```python
from build123d import *

# Parameters (mm, degrees)
SKETCH1_W           = 147.32
SKETCH1_H           = 93.98
SKETCH1_W_2         = 139.7
SKETCH1_H_2         = 86.36
BOSS_EXTRUDE1_DEPTH = 30.48
SKETCH2_W           = 147.32
SKETCH2_H           = 93.98
BOSS_EXTRUDE2_DEPTH = 3.81
FILLET1_R           = 7.62
FILLET2_R           = 5.08
CUT_EXTRUDE2_REACH  = 95.86
SKETCH4_W           = 105.5116
SKETCH4_H           = 67.2084
CUT_EXTRUDE3_REACH  = 94.536
SKETCH5_R           = 2.58


with BuildPart() as part:
    # Sketch1 → Boss-Extrude1 (new body)
    with BuildSketch(Plane(origin=(0, 0, 0), x_dir=(1, 0, 0), z_dir=(0, 1, 0))):
        Rectangle(SKETCH1_W, SKETCH1_H)
        Rectangle(SKETCH1_W_2, SKETCH1_H_2, mode=Mode.SUBTRACT)
    extrude(amount=BOSS_EXTRUDE1_DEPTH)

    # Sketch2 → Boss-Extrude2 (add)
    with BuildSketch(Plane(origin=(0, 0, 0), x_dir=(-1, 0, 0), z_dir=(0, -1, 0))):
        Rectangle(SKETCH2_W, SKETCH2_H)
    extrude(amount=BOSS_EXTRUDE2_DEPTH)

    # Fillet1
    fillet1_edges = [part.edges().sort_by_distance(p)[0] for p in [
        (-73.66, 13.335, -46.99),
        (73.66, 13.335, -46.99),
        (73.66, 13.335, 46.99),
        (-73.66, 13.335, 46.99),
    ]]
    fillet(fillet1_edges, radius=FILLET1_R)

    # Fillet2
    fillet2_edges = [part.edges().sort_by_distance(p)[0] for p in [
        (-69.85, 15.24, -43.18),
        (-69.85, 15.24, 43.18),
        (69.85, 15.24, 43.18),
        (69.85, 15.24, -43.18),
    ]]
    fillet(fillet2_edges, radius=FILLET2_R)

    # Sketch4 → Cut-Extrude2 (cut, up to next)
    with BuildSketch(Plane.XZ.offset(3.81), mode=Mode.PRIVATE) as cut_extrude2_sk1:
        Rectangle(SKETCH4_W, SKETCH4_H)
    cut_extrude2_tool1 = extrude(cut_extrude2_sk1.sketch, amount=-CUT_EXTRUDE2_REACH, mode=Mode.PRIVATE) & part.part
    add(cut_extrude2_tool1.solids().sort_by_distance((0, -3.81, 0))[0], mode=Mode.SUBTRACT)

    # Sketch5 → Cut-Extrude3 (cut, up to next)
    with BuildSketch(Plane(origin=(0, 0, 0), x_dir=(1, 0, 0), z_dir=(0, 1, 0)), mode=Mode.PRIVATE) as cut_extrude3_sk1:
        with Locations(Location((-61.0842, -22.2208, 0), (0, 0, 270))):
            Circle(SKETCH5_R)
    cut_extrude3_tool1 = extrude(cut_extrude3_sk1.sketch, amount=-CUT_EXTRUDE3_REACH, mode=Mode.PRIVATE) & part.part
    # Sketch5 → Cut-Extrude3 (cut, up to next)
    with BuildSketch(Plane(origin=(0, 0, 0), x_dir=(1, 0, 0), z_dir=(0, 1, 0)), mode=Mode.PRIVATE) as cut_extrude3_sk2:
        with Locations(Location((61.0958, -22.2208, 0), (0, 0, 270))):
            Circle(SKETCH5_R)
    cut_extrude3_tool2 = extrude(cut_extrude3_sk2.sketch, amount=-CUT_EXTRUDE3_REACH, mode=Mode.PRIVATE) & part.part
    # Sketch5 → Cut-Extrude3 (cut, up to next)
    with BuildSketch(Plane(origin=(0, 0, 0), x_dir=(1, 0, 0), z_dir=(0, 1, 0)), mode=Mode.PRIVATE) as cut_extrude3_sk3:
        with Locations(Location((61.0958, 22.2292, 0), (0, 0, 270))):
            Circle(SKETCH5_R)
    cut_extrude3_tool3 = extrude(cut_extrude3_sk3.sketch, amount=-CUT_EXTRUDE3_REACH, mode=Mode.PRIVATE) & part.part
    # Sketch5 → Cut-Extrude3 (cut, up to next)
    with BuildSketch(Plane(origin=(0, 0, 0), x_dir=(1, 0, 0), z_dir=(0, 1, 0)), mode=Mode.PRIVATE) as cut_extrude3_sk4:
        with Locations(Location((-61.0842, 22.2292, 0), (0, 0, 270))):
            Circle(SKETCH5_R)
    cut_extrude3_tool4 = extrude(cut_extrude3_sk4.sketch, amount=-CUT_EXTRUDE3_REACH, mode=Mode.PRIVATE) & part.part
    add(cut_extrude3_tool1.solids().sort_by_distance((-61.0842, 0, 22.2208))[0], mode=Mode.SUBTRACT)
    add(cut_extrude3_tool2.solids().sort_by_distance((61.0958, 0, 22.2208))[0], mode=Mode.SUBTRACT)
    add(cut_extrude3_tool3.solids().sort_by_distance((61.0958, 0, -22.2292))[0], mode=Mode.SUBTRACT)
    add(cut_extrude3_tool4.solids().sort_by_distance((-61.0842, 0, -22.2292))[0], mode=Mode.SUBTRACT)


solid = part.part
```
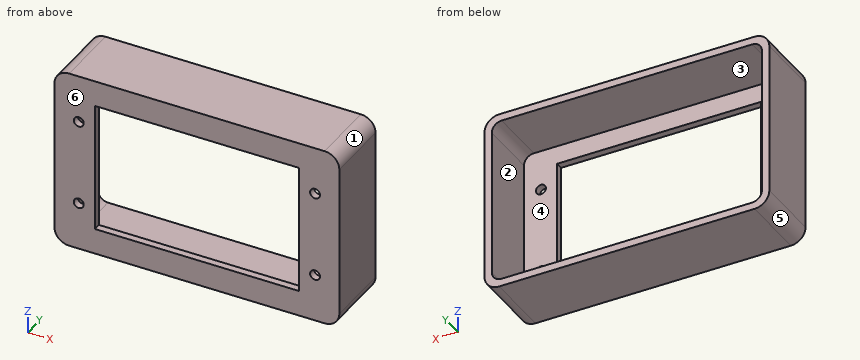
Geometry check sheet. Reference: the model listing, model coordinates, mm. Face numbers are marked on the shaded views. A direction names the side the tool comes from. Give positions to 0.01 mm unless a question says otherwise; leave off trailing zeros. Loops run counter-clockwise (first coordinate to the right, second up) from the corner with the lowest first, then second, coordinate; pieces in that order, holes last. Notation, with made-up numbers: M 74,45 L 118,45 A18 ccw 118,57 Z; hole C 14,62 d1. An arc over 180 degrees is marked long. Write item = value, one per line.
(1) Gauge pin test, flat ends, axial feed: pin 1 Ø5 at (x, z) = (52, 9) entering from +Y; pin 2 Ø4 at (x, z) = (-61.08, -22.23) entering from -Y. Record the tip position at first contact, or that the pin passes through.
Answer below:
pin_1 = 0
pin_2 = through
(2) Sectioned sample at A-A, the plane x = 4.5. Record the cut outline in (y, z).
Answer below:
outline = M -3.81,-46.99 L 30.48,-46.99 L 30.48,-43.18 L 0,-43.18 L 0,-33.6 L -3.81,-33.6 Z; M -3.81,33.6 L 0,33.6 L 0,43.18 L 30.48,43.18 L 30.48,46.99 L -3.81,46.99 Z
(3) Sectioned sample at C-C, the plane z = 4. Record the cut outline in (x, y).
Answer below:
outline = M -73.66,-3.81 L -52.76,-3.81 L -52.76,0 L -69.85,0 L -69.85,30.48 L -73.66,30.48 Z; M 52.76,-3.81 L 73.66,-3.81 L 73.66,30.48 L 69.85,30.48 L 69.85,0 L 52.76,0 Z
(4) Tool access check on the marked faces 1 and 2. Record the directions out of +Z, -Z, +X, -X, +Y, -Y that give a thin tool (end or side, any length) a straight path to the whole face; none if there is none.
Answer below:
face_1 = +Z, +X, +Y, -Y
face_2 = +Y
(5) Release check for a two-part mould opening along X. For the marked faces 3, 4, 5 and 6 record: released by +X, released by -X, zero draft, split by the parting line, or undercut.
Answer below:
face_3 = undercut
face_4 = undercut
face_5 = released by -X
face_6 = zero draft
(6) Material ranges on line 1 (X direction, y = 2, z = -37); line 2 (Z direction, x = 46, y = 27); line 3 (Y direction, x = 66, z = -32.5), recorded low to high. Write a range as [from, to].
Answer below:
line_1 = [-73.66, -69.85], [69.85, 73.66]
line_2 = [-46.99, -43.18], [43.18, 46.99]
line_3 = [-3.81, 0]
(7) Sectioned sample at B-B, the plane y = 4.5. Record the cut outline in (x, z).
Answer below:
outline = M -73.66,-39.37 A7.62 ccw -66.04,-46.99 L 66.04,-46.99 A7.62 ccw 73.66,-39.37 L 73.66,39.37 A7.62 ccw 66.04,46.99 L -66.04,46.99 A7.62 ccw -73.66,39.37 Z; hole M -69.85,-38.1 A5.08 ccw -64.77,-43.18 L 64.77,-43.18 A5.08 ccw 69.85,-38.1 L 69.85,38.1 A5.08 ccw 64.77,43.18 L -64.77,43.18 A5.08 ccw -69.85,38.1 Z
(8) Sectioned sample at D-D, the plane x = 56.5. Record the cut outline in (y, z), plus the area to 3 significant figures.
Answer below:
outline = M -3.81,-46.99 L 30.48,-46.99 L 30.48,-43.18 L 0,-43.18 L 0,43.18 L 30.48,43.18 L 30.48,46.99 L -3.81,46.99 Z
area = 590 mm2
